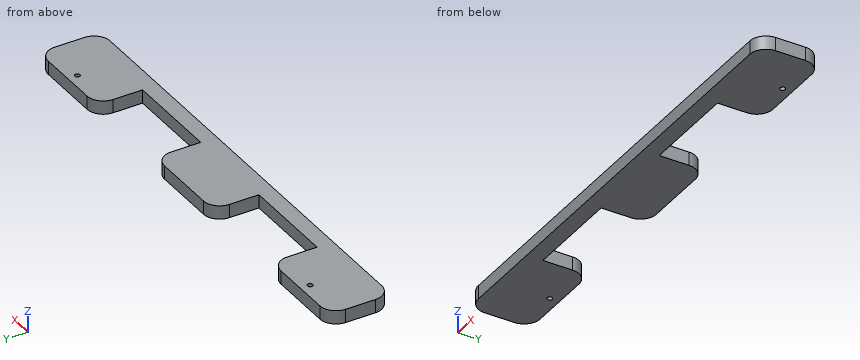
from build123d import *

# Parameters (mm, degrees)
SKETCH1_W           = 190.5
SKETCH1_H           = 24.384
BOSS_EXTRUDE1_DEPTH = 5.334
SKETCH3_W           = 38.1
SKETCH3_H           = 18.034
CUT_EXTRUDE1_DEPTH  = 122.162721385
SKETCH4_R           = 1.016
CUT_EXTRUDE2_DEPTH  = 122.162721385
FILLET1_R           = 6.35


with BuildPart() as part:
    # Sketch1 → Boss-Extrude1 (new body)
    with BuildSketch(Plane.XY):
        with Locations((10.187554582, -47.262819662)):
            Rectangle(SKETCH1_W, SKETCH1_H)
    extrude(amount=BOSS_EXTRUDE1_DEPTH)

    # Sketch3 → Cut-Extrude1 (cut, through all)
    with BuildSketch(Plane.XY.offset(5.334)):
        with Locations((-27.912445418, -44.087819662)):
            Rectangle(SKETCH3_W, SKETCH3_H)
        with Locations((48.287554582, -44.087819662)):
            Rectangle(SKETCH3_W, SKETCH3_H)
    extrude(amount=-CUT_EXTRUDE1_DEPTH, mode=Mode.SUBTRACT)

    # Sketch4 → Cut-Extrude2 (cut, through all)
    with BuildSketch(Plane.XY.offset(5.334)):
        with Locations((-66.012445418, -38.880819662)):
            Circle(SKETCH4_R)
        with Locations(Location((86.387554582, -38.880819662, 0), (0, 0, 180))):
            Circle(SKETCH4_R)
    extrude(amount=-CUT_EXTRUDE2_DEPTH, mode=Mode.SUBTRACT)

    # Fillet1
    fillet1_edges = [part.edges().sort_by_distance(p)[0] for p in [
        (-46.962445418, -35.070819662, 2.667),
        (-8.862445418, -35.070819662, 2.667),
        (29.237554582, -35.070819662, 2.667),
        (67.337554582, -35.070819662, 2.667),
        (-85.062445418, -35.070819662, 2.667),
        (105.437554582, -35.070819662, 2.667),
        (105.437554582, -59.454819662, 2.667),
        (-85.062445418, -59.454819662, 2.667),
    ]]
    fillet(fillet1_edges, radius=FILLET1_R)


solid = part.part
Input: part model. Units: mm. Frame: model coordinates. Coordinates: 2 decimals unless noted, no trailing zeros. Loops run counter-clockwise (first coordinate to the right, second up) from the corner with the lowest first, then second, coordinate; pieces in that order, holes last.
(1) Section D-D on x = -5.5. Return the cut outline in (y, z), then the cut area to 3 significant figures.
(2) Material intervals for probe 1 along X at (y, z) = (-40.75, 4.3); probe 2 along X at (y, z) = (-48.25, 2.3); probe 3 along X at (y, z) = (-38, 1.1), sorted ascending.
(3) Section B-B on z = 3.7. Return the cut outline in (x, y).
(4) First-contact query: pin 1 Ø1.6 at (x, y) = (-66.01, -38.88) entering from +Z; pin 2 Ø1.5 at (y, z) = (-38.5, 2.5) entering from +X; pin 3 Ø2.5 at (x, z) = (47, 3) entering from +Y. Flat tips, straight axial feed; report the tip coordinate or a pass-through.
(5) Section C-C on x = -35. Return the cut outline in (y, z).
(6) Section A-A on y = -46.75. Return the cut outline in (x, z).
Data:
1. outline: (-59.45, 0) - (-35.82, 0) - (-35.82, 5.33) - (-59.45, 5.33) - close
1. area: 126 mm2
2. probe 1: x = -85.03 to -47, -8.83 to 29.2, 67.37 to 105.4
2. probe 2: x = -85.06 to -46.96, -8.86 to 29.24, 67.34 to 105.44
2. probe 3: x = -84.06 to -66.52, -65.51 to -47.96, -7.86 to 28.24, 68.34 to 85.88, 86.89 to 104.44
3. outline: (-85.06, -53.1) arc R6.35 ccw to (-78.71, -59.45) - (99.09, -59.45) arc R6.35 ccw to (105.44, -53.1) - (105.44, -41.42) arc R6.35 ccw to (99.09, -35.07) - (73.69, -35.07) arc R6.35 ccw to (67.34, -41.42) - (67.34, -53.1) - (29.24, -53.1) - (29.24, -41.42) arc R6.35 ccw to (22.89, -35.07) - (-2.51, -35.07) arc R6.35 ccw to (-8.86, -41.42) - (-8.86, -53.1) - (-46.96, -53.1) - (-46.96, -41.42) arc R6.35 ccw to (-53.31, -35.07) - (-78.71, -35.07) arc R6.35 ccw to (-85.06, -41.42) - close; hole circle Ø2.03 at (-66.01, -38.88); hole circle Ø2.03 at (86.39, -38.88)
4. pin 1: passes through
4. pin 2: stops at x = 105.05
4. pin 3: stops at y = -53.1
5. outline: (-59.45, 0) - (-53.1, 0) - (-53.1, 5.33) - (-59.45, 5.33) - close
6. outline: (-85.06, 0) - (-46.96, 0) - (-46.96, 5.33) - (-85.06, 5.33) - close; (-8.86, 0) - (29.24, 0) - (29.24, 5.33) - (-8.86, 5.33) - close; (67.34, 0) - (105.44, 0) - (105.44, 5.33) - (67.34, 5.33) - close
